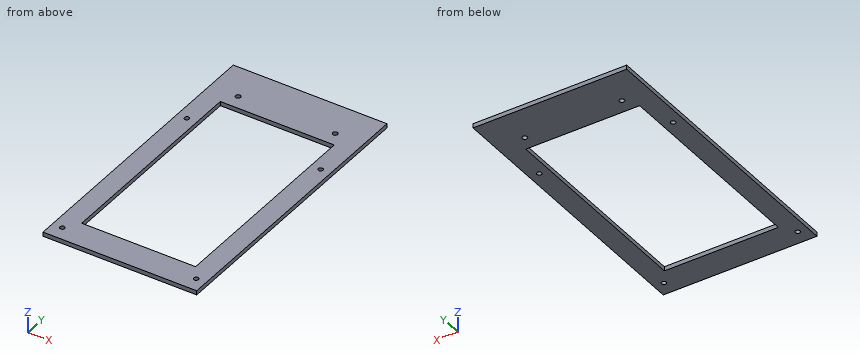
Autodesk Inventor part; units mm, degrees
ref_plane "YZ Plane" through (0, 0, 0) normal (1, 0, 0) x (0, 1, 0)
ref_plane "XZ Plane" through (0, 0, 0) normal (0, 1, 0) x (-1, 0, 0)
ref_plane "XY Plane" through (0, 0, 0) normal (0, 0, 1) x (1, 0, 0)
sketch "Sketch1" plane through (0, 0, 0) normal (0, 0, 1) x (1, 0, 0)
  line L0 (-68.58, -128.7145) -> (68.58, -128.7145)
  line L1 (68.58, -128.7145) -> (68.58, 128.7145)
  line L2 (68.58, 128.7145) -> (-68.58, 128.7145)
  line L3 (-68.58, 128.7145) -> (-68.58, -128.7145)
  line L4 (-68.58, -128.7145) -> (68.58, 128.7145) construction
  line L5 (68.58, -128.7145) -> (-68.58, 128.7145) construction
  point P0 (0, 0)
  dimension "d0" = 137.16
  dimension "d1" = 257.429
extrude "Extrusion1" add sketch "Sketch1" against normal blind 3.81
sketch "Sketch2" plane through (0, 0, 0) normal (0, 0, 1) x (1, 0, 0)
  circle A0 centre (-59.69, 52.5145) radius 2.0955
  line L0 (-68.58, 128.7145) -> (-68.58, -128.7145)
  line L1 (-68.58, 128.7145) -> (68.58, 128.7145)
  circle A1 centre (59.69, 52.5145) radius 2.0955
  line L2 (68.58, -128.7145) -> (68.58, 128.7145)
  circle A2 centre (-59.69, -116.0145) radius 2.0955
  circle A3 centre (59.69, -116.0145) radius 2.0955
  line L3 (-68.58, -128.7145) -> (68.58, -128.7145)
  point P0 (0, 0)
  dimension "d4" = 8.89
  dimension "d5" = 76.2
  dimension "d6" = 76.2
  dimension "d7" = 8.89
  dimension "d8" = 4.191
  dimension "d9" = 12.7
  dimension "d10" = 8.89
  dimension "d11" = 8.89
  dimension "d12" = 12.7
  dimension "d13" = 4.191
  dimension "d21" = 4.191
  dimension "d22" = 4.191
hole "Hole1" at (-59.69, 52.5145, 0) at (59.69, 52.5145, 0) at (-59.69, -116.0145, 0) at (59.69, -116.0145, 0) direction (0, 0, -1) diameter 4.191 end through all
sketch "Sketch5" plane through (0, 0, 0) normal (0, 0, 1) x (1, 0, 0)
  line L0 (-68.58, 128.7145) -> (68.58, 128.7145)
  line L1 (68.58, 128.7145) -> (68.58, -128.7145)
  point P0 (0, 0)
  point P1 (-43.3324, 96.9645)
  point P2 (43.3324, 96.9645)
  dimension "d37" = 31.75
  dimension "d38" = 86.6648
  dimension "d39" = 31.75
  dimension "d40" = 25.2476
hole "Hole2" at (-43.3324, 96.9645, 0) at (43.3324, 96.9645, 0) direction (0, 0, -1) diameter 4.4704 end through all
sketch "battery_buzzer" plane through (0, 0, 0) normal (0, 0, 1) x (1, 0, 0)
  point P0 (0, 0)
sketch "Sketch7" plane through (0, 0, 0) normal (0, 0, 1) x (1, 0, 0)
  line L0 (-50.8, 39.5798) -> (-50.8, -103.3145)
  line L1 (-50.8, -103.3145) -> (50.8, -103.3145)
  line L2 (50.8, -103.3145) -> (50.8, 39.5798)
  line L3 (50.8, 39.5798) -> (50.8, 84.2645)
  line L4 (50.8, 84.2645) -> (-50.8, 84.2645)
  line L5 (-50.8, 84.2645) -> (-50.8, 39.5798)
  line L6 (68.58, -128.7145) -> (68.58, 128.7145)
  line L7 (-68.58, 128.7145) -> (-68.58, -128.7145)
  line L8 (68.58, -128.7145) -> (-68.58, -128.7145)
  line L9 (68.58, 128.7145) -> (-68.58, 128.7145)
  point P0 (0, 0)
  dimension "d48" = 17.78
  dimension "d49" = 17.78
  dimension "d50" = 25.4
  dimension "d51" = 44.45
extrude "Extrusion3" cut sketch "Sketch7" against normal blind 3.81 contours L5 L4 L3 L2 L1 L0
Verification items for the finished model (mm, model axes). Round coordinates to 2 decimals unless told otherwise and drop trailing zeros. Write each loop counter-clockwise with the first axis right and the second up, starting at its lowest first coordinate (ties: lowest second). Pieces come first, ordered by that corner, then holes.
1. Section check B-B on y = -56.5. Enter the section's corners in (x, z).
2. Section check C-C on z = -1.9. Enter the section's corners in (x, y).
3. Scan lines: L1, parallel to Y at x = 59.69, z = -2.9; L2, parallel to Y at x = 43.5, z = -2.7; L3, parallel to Y at x = 13.5, z = -1.7. Record each from-to range of solid material in increasing order.
4. Gauge pin test, flat end, axial feed: P1, Ø2.5, axis at x = -43.33, y = 96.96, coming from the -Z side. Record the tip position at first contact, or that the pin passes through.
5. Section check A-A on x = 18. Enter the section's corners in (y, z), plus the area to 3 significant figures.
Answer:
1. outline: (-68.58, -3.81) - (-50.8, -3.81) - (-50.8, 0) - (-68.58, 0) - close; (50.8, -3.81) - (68.58, -3.81) - (68.58, 0) - (50.8, 0) - close
2. outline: (-68.58, -128.71) - (68.58, -128.71) - (68.58, 128.71) - (-68.58, 128.71) - close; hole circle Ø4.19 at (-59.69, -116.01); hole circle Ø4.19 at (-59.69, 52.51); hole (-50.8, -103.31) - (50.8, -103.31) - (50.8, 84.26) - (-50.8, 84.26) - close; hole circle Ø4.47 at (-43.33, 96.96); hole circle Ø4.47 at (43.33, 96.96); hole circle Ø4.19 at (59.69, -116.01); hole circle Ø4.19 at (59.69, 52.51)
3. L1: y = -128.71 to -118.11, -113.92 to 50.42, 54.61 to 128.71
3. L2: y = -128.71 to -103.31, 84.26 to 94.74, 99.19 to 128.71
3. L3: y = -128.71 to -103.31, 84.26 to 128.71
4. P1: passes through
5. outline: (-128.71, -3.81) - (-103.31, -3.81) - (-103.31, 0) - (-128.71, 0) - close; (84.26, -3.81) - (128.71, -3.81) - (128.71, 0) - (84.26, 0) - close
5. area: 266 mm2
